Input: part model. Units: mm. Frame: model coordinates. A direction names the side the tool comes from. Coordinates: 2 decimals unless noted, no trailing zeros. Write each loop counter-clockwise with the first axis right and the second up, starting at its lowest first coordinate (ties: lowest second). Pieces come first, ordered by that corner, then holes. Notation, with made-up numbers: M 16,13 L 63,13 A30 ccw 63,39 Z; hole C 3.25,79 d7. An arc over 180 degrees is marked long. Use CSV: the item, a comma, the result in double quotes.
```python
from build123d import *

# Parameters (mm, degrees)
F0_R     = 3.175
F1_DEPTH = 3.048


with BuildPart() as f1:
    # F0 (on Front) → F1 (new body)
    with BuildSketch(Plane.XZ):
        with BuildLine():
            ThreePointArc((-2.38125, 105.077459), (5.832847, 106.769826), (9.525, 114.3))
            ThreePointArc((9.525, 114.3), (9.506305, 114.896483), (9.450293, 115.490625))
            ThreePointArc((9.450293, 115.490625), (-0.596483, 123.806305), (-9.525, 114.3))
            ThreePointArc((-9.525, 114.3), (-7.530174, 108.467153), (-2.38125, 105.077459))
        make_face()
        with Locations((0, 114.3)):
            Circle(F0_R, mode=Mode.SUBTRACT)
        with BuildLine():
            ThreePointArc((9.450293, 115.490625), (9.506305, 114.896483), (9.525, 114.3))
            ThreePointArc((9.525, 114.3), (5.832847, 106.769826), (-2.38125, 105.077459))
            ThreePointArc((-2.38125, 105.077459), (-7.530174, 108.467153), (-9.525, 114.3))
            Line((-9.525, 114.3), (-15.747457, 65.508289))
            ThreePointArc((-15.747457, 65.508289), (0.012053, 79.374995), (15.750488, 65.484375))
            Line((15.750488, 65.484375), (9.450293, 115.490625))
        make_face()
        with BuildLine():
            ThreePointArc((0, 102.003278), (-5.685058, 100.058995), (-2.38125, 105.077459))
            ThreePointArc((-2.38125, 105.077459), (-0.664942, 103.947561), (0, 102.003278))
        make_face(mode=Mode.SUBTRACT)
        with BuildLine():
            ThreePointArc((15.875, 63.5), (15.843841, 64.494139), (15.750488, 65.484375))
            ThreePointArc((15.750488, 65.484375), (0.012053, 79.374995), (-15.747457, 65.508289))
            ThreePointArc((-15.747457, 65.508289), (-15.873668, 63.705667), (-15.794203, 61.90038))
            ThreePointArc((-15.794203, 61.90038), (-0.193615, 47.626181), (15.750488, 61.515625))
            ThreePointArc((15.750488, 61.515625), (15.843841, 62.505861), (15.875, 63.5))
        make_face()
        with Locations((0, 63.5)):
            Circle(F0_R, mode=Mode.SUBTRACT)
        with BuildLine():
            ThreePointArc((15.750488, 61.515625), (-0.193615, 47.626181), (-15.794203, 61.90038))
            Line((-15.794203, 61.90038), (-9.525, 0))
            ThreePointArc((-9.525, 0), (0, 9.525), (9.525, 0))
            ThreePointArc((9.525, 0), (8.392738, -4.504173), (5.265142, -7.9375))
            Line((5.265142, -7.9375), (31.75, -7.9375))
            ThreePointArc((31.75, -7.9375), (23.814982, 0.1985), (32.146875, 7.927572))
            Line((32.146875, 7.927572), (17.706028, 8.650519))
            ThreePointArc((17.706028, 8.650519), (12.011247, 11.482969), (10.215693, 17.58455))
            Line((10.215693, 17.58455), (15.750488, 61.515625))
        make_face()
        with BuildLine():
            ThreePointArc((9.525, 0), (0, 9.525), (-9.525, 0))
            ThreePointArc((-9.525, 0), (-4.504173, -8.392738), (5.265142, -7.9375))
            ThreePointArc((5.265142, -7.9375), (8.392738, -4.504173), (9.525, 0))
        make_face()
        Circle(F0_R, mode=Mode.SUBTRACT)
        with BuildLine():
            ThreePointArc((32.146875, 7.927572), (23.814982, 0.1985), (31.75, -7.9375))
            ThreePointArc((31.75, -7.9375), (37.36266, -5.61266), (39.6875, 0))
            ThreePointArc((39.6875, 0), (37.501265, 5.470544), (32.146875, 7.927572))
        make_face()
        with Locations((31.75, 0)):
            Circle(F0_R, mode=Mode.SUBTRACT)
    extrude(amount=F1_DEPTH)


solid = f1.part
```
1. Material intervals for line 1 (Z direction, x = -0.5, y = -0.5); line 2 (Z direction, x = -6, y = -1.1); line 3 (X direction, y = -1.15, z = 112), sorted ascending. Write a range as [from, to].
Resolved:
line 1,"z = [-9.51, -3.14], [3.14, 60.36], [66.64, 100.29], [103.71, 111.16], [117.44, 123.81]"
line 2,"z = [-7.4, 100.55], [103.45, 121.7]"
line 3,"x = [-9.82, -2.19], [2.19, 9.89]"
2. Section A-A (y = -0.85). State how many separate pieces and enclosed holes the cut face has, then the cut area to 3 significant figures.
Resolved:
separate pieces,"1"
enclosed holes,"5"
area,"3,500 mm^2"
3. Section B-B (z = 58.5). Return loops of the section in (x, y), then the cut area to 3 significant figures.
Resolved:
outline,"M -15.45,-3.05 L 15.37,-3.05 L 15.37,0 L -15.45,0 Z"
area,"93.9 mm^2"
4. Mould query, pull axis X, two halves, no side actions, for faces 1 (the flat face through (5, 0, 43)), 2 (the cylindrical face through (12.071, -1.503, 11.413)), 3 (the cylindrical face through (-0.396, -1.503, 123.817)), 4 (the cylindrical face through (1.707, -1.503, 66.177)). Classes: pulls with the +X half, pulls with the -X half, needs draft (parallel to the pull), parting line crosses it, or undercut.
Resolved:
face 1,"needs draft"
face 2,"pulls with the +X half"
face 3,"parting line crosses it"
face 4,"undercut"
5. Section C-C (x = 22). Return loops of the section in (y, z), then the cut area to 3 significant figures.
Resolved:
outline,"M -3.05,-7.94 L 0,-7.94 L 0,8.44 L -3.05,8.44 Z"
area,"49.9 mm^2"
6. Contact query for a flat-ended pin moving along its axis: pin 1 Ø1 at (x, y) = (19.5, -2.5) entering from -Z. Output: stop coordinate, or through.
Resolved:
pin 1,"stops at z = -7.94"
7. Access query for faces 5 (the flat face through (5, -3.048, 43)), 6 (the flat face through (18, -2, -7.938)), 7 (the flat face through (12.944, -1.503, 39.243)). Directions: +Z, -Z, +X, -X, +Y, -Y. A direction counts if a zero-diameter tool reaches every point of the face in a straight line with its end or side. Return the directions, or none.
Resolved:
face 5,"+Z, -Z, +X, -X, -Y"
face 6,"-Z, +X, +Y, -Y"
face 7,"+X, +Y, -Y"
